```python
from build123d import *

# Parameters (mm, degrees)
ESQUISSE1_R        = 2.5
BOSS_EXTRU_1_DEPTH = 10
CONG_1_R           = 2


with BuildPart() as part:
    # Esquisse1 → Boss.-Extru.1 (new body)
    with BuildSketch(Plane.XY):
        with BuildLine():
            Line((0.1, 14), (0, 14))
            Line((0, 14), (0, 28))
            Line((0, 28), (-13, 28))
            Line((-13, 28), (-13, 38))
            Line((-13, 38), (-23, 38))
            Line((-23, 38), (-23, -16.88168582))
            Line((-23, -16.88168582), (-13, -16.88168582))
            Line((-13, -16.88168582), (-13, -6.88168582))
            Line((-13, -6.88168582), (0.1, -6.88168582))
            Line((0.1, -6.88168582), (0.1, -14))
            ThreePointArc((0.1, -14), (0.363603897, -14.636396103), (1, -14.9))
            Line((1, -14.9), (2.585786438, -14.9))
            ThreePointArc((2.585786438, -14.9), (2.930201527, -14.831491579), (3.222182541, -14.636396103))
            Line((3.222182541, -14.636396103), (9.586143571, -8.272435072))
            ThreePointArc((9.586143571, -8.272435072), (9.849747468, -7.636038969), (9.586143571, -6.999642866))
            Line((9.586143571, -6.999642866), (8.87903679, -6.292536085))
            ThreePointArc((8.87903679, -6.292536085), (8.242640687, -6.028932188), (7.606244584, -6.292536085))
            Line((7.606244584, -6.292536085), (4.777817459, -9.12096321))
            ThreePointArc((4.777817459, -9.12096321), (3.579048224, -9.359413236), (2.9, -8.343145751))
            Line((2.9, -8.343145751), (2.9, 8.343145751))
            ThreePointArc((2.9, 8.343145751), (3.579048224, 9.359413236), (4.777817459, 9.12096321))
            Line((4.777817459, 9.12096321), (7.606244584, 6.292536085))
            ThreePointArc((7.606244584, 6.292536085), (8.242640687, 6.028932188), (8.87903679, 6.292536085))
            Line((8.87903679, 6.292536085), (9.586143571, 6.999642866))
            ThreePointArc((9.586143571, 6.999642866), (9.849747468, 7.636038969), (9.586143571, 8.272435072))
            Line((9.586143571, 8.272435072), (3.222182541, 14.636396103))
            ThreePointArc((3.222182541, 14.636396103), (2.930201527, 14.831491579), (2.585786438, 14.9))
            Line((2.585786438, 14.9), (1, 14.9))
            ThreePointArc((1, 14.9), (0.363603897, 14.636396103), (0.1, 14))
        make_face()
        with Locations((-17.5, 7.5)):
            Circle(ESQUISSE1_R, mode=Mode.SUBTRACT)
        with Locations((-17.5, -7.5)):
            Circle(ESQUISSE1_R, mode=Mode.SUBTRACT)
    extrude(amount=BOSS_EXTRU_1_DEPTH)

    # Congé1
    cong_1_edges = [part.edges().sort_by_distance(p)[0] for p in [
        (-13, -6.88168582, 5),
        (-13, -16.88168582, 5),
        (-23, -16.88168582, 5),
        (-23, 38, 5),
        (-13, 38, 5),
        (-13, 28, 5),
        (0, 28, 5),
    ]]
    fillet(cong_1_edges, radius=CONG_1_R)


solid = part.part
```
Could you check a few things on this model? Use its own coordinates, in mm. A direction names the side the tool comes from. Coordinates: 2 decimals unless noted, no trailing zeros. Loops run counter-clockwise (first coordinate to the right, second up) from the corner with the lowest first, then second, coordinate; pieces in that order, holes last.
1) Thinking about a two-plate mould opening in X: for faces 5 (the face through (-18, -16.882, 5)), 6 (the face through (6.2, 7.7, 4.9)), 7 (the face through (-12.4, 28.57, 5.07)), which applies, released by +X, released by -X, zero draft, split by the parting line, or undercut?
Reported:
face 5: zero draft
face 6: undercut
face 7: released by +X
2) Will these pins go through, and if not, where does the flat tip stop? pin 1 Ø3 at (y, z) = (-12, 4.5) entering from +X; pin 2 Ø5 at (x, z) = (1.5, 8) entering from -Y; pin 3 Ø3 at (x, z) = (-7, 7) entering from -Y; pin 4 Ø4.5 at (x, y) = (-17.5, -7.5) entering from -Z.
Reported:
pin 1: stops at x = 7.36
pin 2: stops at y = -14.9
pin 3: stops at y = -6.88
pin 4: passes through
3) Imagine slicing it at D-D (x = -9). List the corners of the cut face in (y, z) for me.
Reported:
outline: (-6.88, 0) - (28, 0) - (28, 10) - (-6.88, 10) - close
4) Imagine slicing it at A-A (x = -17.5). List the corners of the cut face in (y, z) for me.
Reported:
outline: (-16.88, 0) - (-10, 0) - (-10, 10) - (-16.88, 10) - close; (-5, 0) - (5, 0) - (5, 10) - (-5, 10) - close; (10, 0) - (38, 0) - (38, 10) - (10, 10) - close
5) Which directions (+Z, -Z, +X, -X, +Y, -Y) give clear straight access to the entire face, cutting with the end or side of a thin tool? Please do faces 1 (the face through (6.2, -7.7, 4.9)), 2 (the face through (-13, 33, 5)), 3 (the face through (2, -14.9, 5)), 4 (the face through (-6, -6.882, 5)).
Reported:
face 1: +Z, -Z
face 2: +Z, -Z, +X, +Y
face 3: +Z, -Z, +X, -Y
face 4: +Z, -Z, -Y
6) Imagine slicing it at B-B (z = 3.5). State how many separate pieces and enclosed holes the cut face has, and give its area (3 significant figures).
Reported:
separate pieces: 1
enclosed holes: 2
area: 1,100 mm2
7) Please list where these lines run through material, in increasing order: line 1 along Y through (x, z) = (-17.5, 4.5); line 2 along X through (y, z) = (17, 5); line 3 along Y through (x, z) = (-9.5, 6.5).
Reported:
line 1: y = -16.88 to -10, -5 to 5, 10 to 38
line 2: x = -23 to 0
line 3: y = -6.88 to 28
8) Imagine slicing it at C-C (y = 22.5). List the corners of the cut face in (x, z) for me, and give its area (3 significant figures).
Reported:
outline: (-23, 0) - (0, 0) - (0, 10) - (-23, 10) - close
area: 230 mm2
